Input: dimensioned drawing with shaded views. Units: mm. Origin: part minimum x, y, z. A direction names the side the tool comes from. Round coordinates to 2 decimals unless told otherwise and drop trailing zeros. Loops run counter-clockwise (first coordinate to the right, second up) from the corner with the lowest first, then second, coordinate; pieces in that order, holes last. Notation, with made-up numbers: (44, 11.25) - (72, 11.25) arc R17 ccw to (72, 36.25) - close; hole circle Ø7 at (17, 28). An arc over 180 degrees is marked (long way). Answer as a JSON object with one key per item and string values. Group by question number.
Item 1: Reachability of the marked faces 4 and 5 from +Z, -Z, +X, -X, +Y, -Y: full face, straight path, thin tool, end or side. Return the list, or none.
Item 2: Section C-C (y = 4.1). Return the cut outline in (x, z), plus the area to 3 significant figures.
Item 3: First-contact query: pin 1 (2.5 mm diameter, centred on x = 3.25, z = 10.25, fed in from -Y); pin 2 (2 mm diameter, centred on x = 8.5, y = 2.5, fed in from +Z); pin 3 (3 mm diameter, centred on x = 11.5, z = 9, fed in from -Y); pin 4 (3 mm diameter, centred on x = 18, y = 4.5, fed in from +Z). Flat tips, straight axial feed; report the tip coordinate or a pass-through.
Item 4: Section D-D (z = 17.25). Return the cut outline in (x, y), plus the area to 4 significant figures.
Item 5: Draft query along Z for the marked faces 1, 2 and 3. Return one class per face: released by +Z, released by -Z, zero draft, split by the parting line, or undercut.
Item 6: Line query: line 1 (Z direction, x = 10.25, y = 3.95); line 2 (Z direction, x = 10.25, y = 2.15). Output: solid intervals per line, ascending.
Item 7: Section B-B (z = 10.5). Return the cut outline in (x, y), plus the area to 3 significant figures.
Item 8: Section A-A (x = 10.25). Return the cut outline in (y, z).
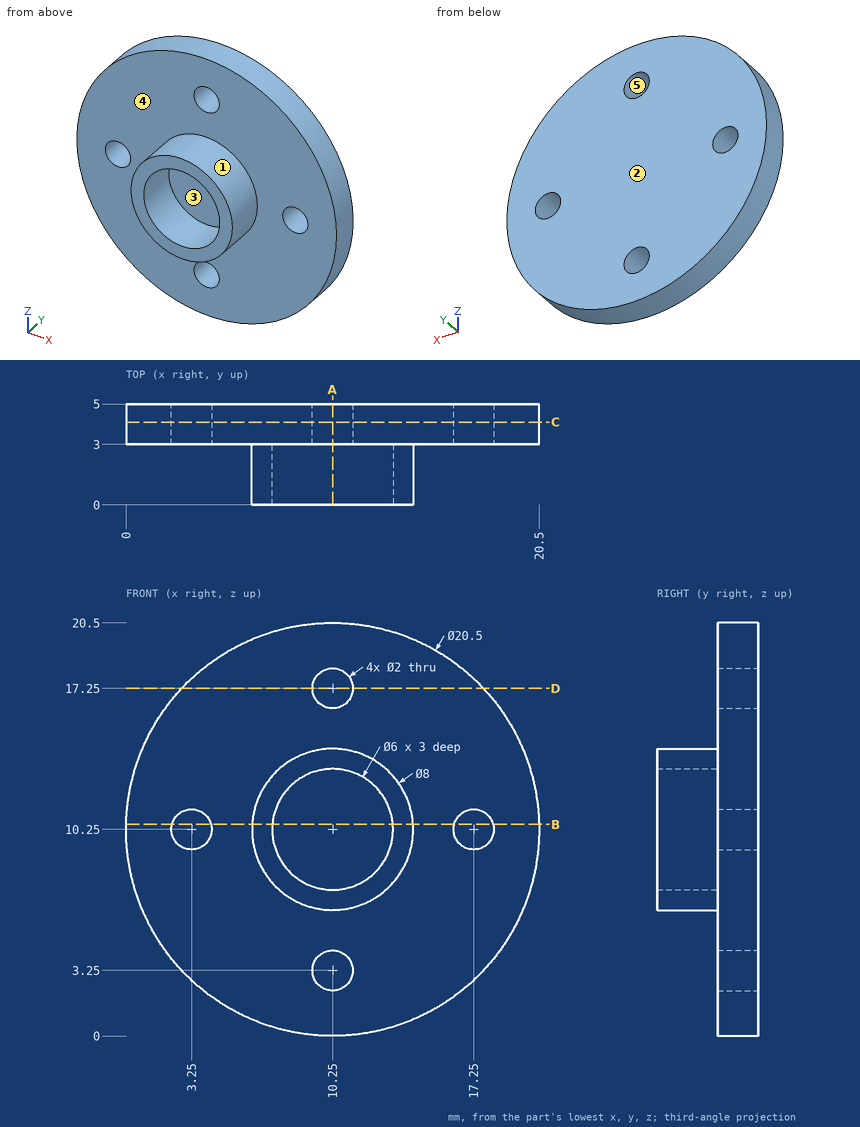
Values:
{
 "1": {"face 4": "-Y", "face 5": "+Y, -Y"},
 "2": {"outline": "circle Ø20.5 at (10.25, 10.25); hole circle Ø2 at (3.25, 10.25); hole circle Ø2 at (10.25, 3.25); hole circle Ø2 at (10.25, 17.25); hole circle Ø2 at (17.25, 10.25)", "area": "317 mm^2"},
 "3": {"pin 1": "stops at y = 3", "pin 2": "stops at z = 20.46", "pin 3": "stops at y = 0", "pin 4": "stops at z = 18.37"},
 "4": {"outline": "(2.76, 3) - (9.25, 3) - (9.25, 5) - (2.76, 5) - close; (11.25, 3) - (17.74, 3) - (17.74, 5) - (11.25, 5) - close", "area": "25.95 mm^2"},
 "5": {"face 1": "split by the parting line", "face 2": "zero draft", "face 3": "undercut"},
 "6": {"line 1": "z = 0 to 2.25, 4.25 to 16.25, 18.25 to 20.5", "line 2": "z = 6.25 to 7.25, 13.25 to 14.25"},
 "7": {"outline": "(0, 3) - (2.28, 3) - (2.28, 5) - (0, 5) - close; (4.22, 3) - (6.26, 3) - (6.26, 0) - (7.26, 0) - (7.26, 3) - (13.24, 3) - (13.24, 0) - (14.24, 0) - (14.24, 3) - (16.28, 3) - (16.28, 5) - (4.22, 5) - close; (18.22, 3) - (20.5, 3) - (20.5, 5) - (18.22, 5) - close", "area": "39.3 mm^2"},
 "8": {"outline": "(0, 6.25) - (3, 6.25) - (3, 4.25) - (5, 4.25) - (5, 16.25) - (3, 16.25) - (3, 14.25) - (0, 14.25) - (0, 13.25) - (3, 13.25) - (3, 7.25) - (0, 7.25) - close; (3, 0) - (5, 0) - (5, 2.25) - (3, 2.25) - close; (3, 18.25) - (5, 18.25) - (5, 20.5) - (3, 20.5) - close"}
}
